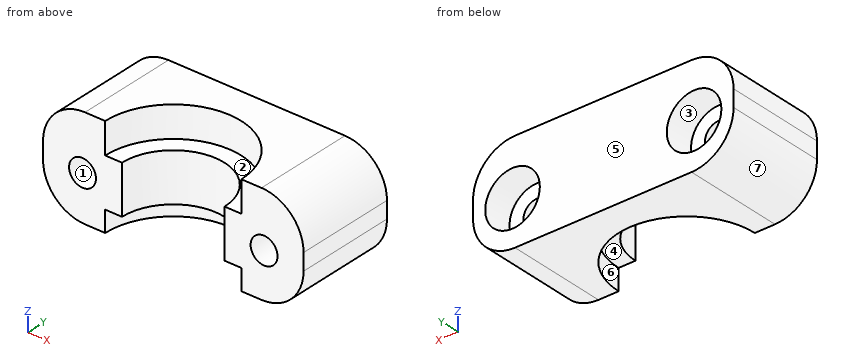
from build123d import *

# Parameters (mm, degrees)
F1_DEPTH = 3.7
F3_DEPTH = 5.8
F5_DEPTH = 2.5
F6_R     = 1.6
F7_DEPTH = 12.001
F8_R     = 3.25
F9_DEPTH = 3.5
F10_R    = 5


with BuildPart() as f1:
    # F0 (on Top) → F1 (new body)
    with BuildSketch(Plane.XY):
        with BuildLine():
            Line((15.5, 12), (-15.5, 12))
            Line((-15.5, 12), (-15.5, 0))
            Line((-15.5, 0), (-8.1, 0))
            ThreePointArc((-8.1, 0), (0, 8.1), (8.1, 0))
            Line((8.1, 0), (15.5, 0))
            Line((15.5, 0), (15.5, 12))
        make_face()
    extrude(amount=-F1_DEPTH)

    # F2 (on face) → F3 (join)
    with BuildSketch(Plane(origin=(0, 0, -3.7), x_dir=(1, 0, 0), z_dir=(0, 0, -1))):
        with BuildLine():
            Line((0, -12), (15.5, -12))
            Line((15.5, -12), (15.5, 0))
            Line((15.5, 0), (6.1, 0))
            ThreePointArc((6.1, 0), (0, -6.1), (-6.1, 0))
            Line((-6.1, 0), (-8.1, 0))
            Line((-8.1, 0), (-15.5, 0))
            Line((-15.5, 0), (-15.5, -12))
            Line((-15.5, -12), (0, -12))
        make_face()
    extrude(amount=F3_DEPTH)

    # F4 (on face) → F5 (join)
    with BuildSketch(Plane(origin=(0, 0, -9.5), x_dir=(1, 0, 0), z_dir=(0, 0, -1))):
        with BuildLine():
            Line((15.5, 0), (8.1, 0))
            ThreePointArc((8.1, 0), (0, -8.1), (-8.1, 0))
            Line((-8.1, 0), (-15.5, 0))
            Line((-15.5, 0), (-15.5, -12))
            Line((-15.5, -12), (15.5, -12))
            Line((15.5, -12), (15.5, 0))
        make_face()
    extrude(amount=F5_DEPTH)

    # F6 (on face) → F7 (cut, through all)
    with BuildSketch(Plane.XZ):
        with Locations((-10.8, -6.6)):
            Circle(F6_R)
        with Locations((10.8, -6.6)):
            Circle(F6_R)
    extrude(amount=-F7_DEPTH, mode=Mode.SUBTRACT)

    # F8 (on face) → F9 (cut)
    with BuildSketch(Plane(origin=(0, 12, 0), x_dir=(-1, 0, 0), z_dir=(0, 1, 0))):
        with Locations((-10.8, -6.6)):
            Circle(F8_R)
        with Locations((10.8, -6.6)):
            Circle(F8_R)
    extrude(amount=-F9_DEPTH, mode=Mode.SUBTRACT)

    # F10
    f10_edges = [f1.edges().sort_by_distance(p)[0] for p in [
        (15.5, 6, 0),
        (15.5, 6, -12),
        (-15.5, 6, 0),
        (-15.5, 6, -12),
    ]]
    fillet(f10_edges, radius=F10_R)


solid = f1.part
Design review of the part built by this model. Coordinates are the model's own, in mm. Face numbers are marked on the shaded views. A direction names the side the tool comes from. Coordinates: 2 decimals unless noted, no trailing zeros. Loops run counter-clockwise (first coordinate to the right, second up) from the corner with the lowest first, then second, coordinate; pieces in that order, holes last. Notation, with made-up numbers: (-31, 12.5) - (-10, 12.5) arc R21 ccw to (-10, 48.5) - close; hole circle Ø8 at (-29, 22.5). An arc over 180 degrees is marked (long way). Use CSV: the item, a comma, the result in double quotes. Start each with the question number.
1. For the marked faces 1, 2, 3 and 4, list the 3-axis set-ups (+Z, -Z, +X, -X, +Y, -Y) from which the entire face can be reached by the end or side of a thin tool; tool diameter is ignored.
2. Add section C-C on z = -6.6. Give the boundary of the cut face in (x, y).
3. Add section B-B on y = 4.25. Give the boundary of the cut face in (x, z), plus the area to 3 significant figures.
4. To check wall thickness, follow probe 1 along Z at (x, y) = (10.8, 2.5); probe 2 along Y at (x, z) = (0, -3); probe 3 along Z at (x, y) = (-10.8, 9.3). State the ranges of each line that lie inside material, in increasing order.
5. Clearance check with flat-ended pins moving along their axes: pin 1 (4 mm diameter, centred on x = 10.8, z = -6.6, fed in from +Y); pin 2 (6.5 mm diameter, centred on x = 1, y = 4, fed in from -Z); pin 3 (2.5 mm diameter, centred on x = -10.8, z = -6.6, fed in from +Y); pin 4 (6.5 mm diameter, centred on x = 2.5, y = 3.5, fed in from +Z). State where each tip first meets the part, or that it passes through.
6. Add section D-D on x = 0. Give the boundary of the cut face in (y, z), plus the area to 3 significant figures.
7. Mouldability with a two-part tool opening along X and no side actions: class the marked faces 5, 6 and 7 as released by +X, released by -X, zero draft, split by the parting line, or undercut.
8. Add section A-A on y = 10.75. Give the boundary of the cut face in (x, z).
Resolved:
1,face 1,"+Y, -Y"
1,face 2,"+Z, -Y"
1,face 3,"+Y"
1,face 4,"-Z, -Y"
2,outline,"(-15.5, 0) - (-12.4, 0) - (-12.4, 8.5) - (-14.05, 8.5) - (-14.05, 12) - (-15.5, 12) - close; (-9.2, 0) - (-6.1, 0) arc R6.1 cw to (6.1, 0) - (9.2, 0) - (9.2, 8.5) - (7.55, 8.5) - (7.55, 12) - (-7.55, 12) - (-7.55, 8.5) - (-9.2, 8.5) - close; (12.4, 0) - (15.5, 0) - (15.5, 12) - (14.05, 12) - (14.05, 8.5) - (12.4, 8.5) - close"
3,outline,"(-15.5, -7) arc R5 ccw to (-10.5, -12) - (-6.9, -12) - (-6.9, -9.5) - (-4.38, -9.5) - (-4.38, -3.7) - (-6.9, -3.7) - (-6.9, 0) - (-10.5, 0) arc R5 ccw to (-15.5, -5) - close; (4.38, -9.5) - (6.9, -9.5) - (6.9, -12) - (10.5, -12) arc R5 ccw to (15.5, -7) - (15.5, -5) arc R5 ccw to (10.5, 0) - (6.9, 0) - (6.9, -3.7) - (4.38, -3.7) - close; hole circle Ø3.2 at (-10.8, -6.6); hole circle Ø3.2 at (10.8, -6.6)"
3,area,"198 mm2"
4,probe 1,"-11.99 to -8.2, -5 to -0.01"
4,probe 2,"8.1 to 12"
4,probe 3,"-11.99 to -9.85, -3.35 to -0.01"
5,pin 1,"y = 8.5"
5,pin 2,"z = -9.5"
5,pin 3,"through"
5,pin 4,"z = -3.7"
6,outline,"(6.1, -9.5) - (8.1, -9.5) - (8.1, -12) - (12, -12) - (12, 0) - (8.1, 0) - (8.1, -3.7) - (6.1, -3.7) - close"
6,area,"58.4 mm2"
7,face 5,"zero draft"
7,face 6,"undercut"
7,face 7,"released by -X"
8,outline,"(-15.5, -7) arc R5 ccw to (-10.5, -12) - (10.5, -12) arc R5 ccw to (15.5, -7) - (15.5, -5) arc R5 ccw to (10.5, 0) - (-10.5, 0) arc R5 ccw to (-15.5, -5) - close; hole circle Ø6.5 at (-10.8, -6.6); hole circle Ø6.5 at (10.8, -6.6)"
